The model under review builds one solid part; all positions refer to its coordinate system, in mm. Face numbers are marked on the shaded views. Round coordinates to 2 decimals unless told otherwise and drop trailing zeros. Loops run counter-clockwise (first coordinate to the right, second up) from the corner with the lowest first, then second, coordinate; pieces in that order, holes last. Notation, with made-up numbers: M 35.25,3.5 L 62.25,3.5 A35 cw 62.25,42.5 Z; hole C -7,-30.75 d2. An arc over 180 degrees is marked long. One line per question, with ' | ' between items.
from build123d import *

# Parameters (mm, degrees)
ESBO_O1_R                = 5.25
RESSALTO_EXTRUS_O1_DEPTH = 28.2
ESBO_O1_5_R              = 5
RESSALTO_EXTRUS_O3_DEPTH = 22
RESSALTO_EXTRUS_O4_DEPTH = 27.5
RESSALTO_EXTRUS_O5_DEPTH = 27.5
CORTE_EXTRUS_O3_DEPTH    = 153.972464187
ESBO_O3_R                = 2
CORTE_EXTRUS_O4_DEPTH    = 161.384600668


with BuildPart() as part:
    # Esbo_o1 → Ressalto-extrus_o1 (new, symmetric)
    with BuildSketch(Plane.XY):
        Circle(ESBO_O1_R)
    extrude(amount=RESSALTO_EXTRUS_O1_DEPTH, both=True)

    # Esbo_o1_7 → Ressalto-extrus_o4 (add, symmetric)
    with BuildSketch(Plane.XY):
        with BuildLine():
            Line((60, 5.000779295), (1.598344907, 5.000779295))
            ThreePointArc((1.598344907, 5.000779295), (4.239918087, 3.096061146), (5.25, 0))
            ThreePointArc((5.25, 0), (4.239918087, -3.096061146), (1.598344907, -5.000779295))
            Line((1.598344907, -5.000779295), (60, -5.000779295))
            Line((60, -5.000779295), (60, 5.000779295))
        make_face()
    extrude(amount=RESSALTO_EXTRUS_O4_DEPTH, both=True)



with BuildPart() as body_2:
    # Esbo_o1_5 → Ressalto-extrus_o3 (new, symmetric)
    with BuildSketch(Plane.XY):
        with Locations((145, 1.500779295)):
            Circle(ESBO_O1_5_R)
    extrude(amount=RESSALTO_EXTRUS_O3_DEPTH, both=True)


with BuildPart() as part_1:
    add(part.part)

    add(body_2.part)  # Ressalto-extrus_o5 merges body 2
    # Esbo_o1_8 → Ressalto-extrus_o5 (add, symmetric)
    with BuildSketch(Plane.XY):
        with BuildLine():
            Line((144.911732622, 6.500000121), (60, 5.000779295))
            Line((60, 5.000779295), (60, -5.000779295))
            Line((60, -5.000779295), (145.088267378, -3.498441531))
            ThreePointArc((145.088267378, -3.498441531), (140.000779174, 1.412511917), (144.911732622, 6.500000121))
        make_face()
    extrude(amount=RESSALTO_EXTRUS_O5_DEPTH, both=True)

    # Esbo_o2 → Corte-extrus_o3 (cut, through all)
    with BuildSketch(Plane(origin=(-0.069568666, 3.940177355, 0), x_dir=(0.9998441652583014, 0.01765347554818762, 0), z_dir=(-0.017653475548187615, 0.9998441652583013, 0))):
        Polygon((60.078931051, -27.5), (145.003897933, -22), (145.003897933, -27.5), align=None)
        Polygon((60.078931051, 27.5), (145.003897933, 22), (145.003897933, 27.5), align=None)
    extrude(amount=-CORTE_EXTRUS_O3_DEPTH, mode=Mode.SUBTRACT)

    # Esbo_o3 → Corte-extrus_o4 (cut, through all)
    with BuildSketch(Plane.XY.offset(28.2)):
        Circle(ESBO_O3_R)
    extrude(amount=-CORTE_EXTRUS_O4_DEPTH, mode=Mode.SUBTRACT)


solid = part_1.part
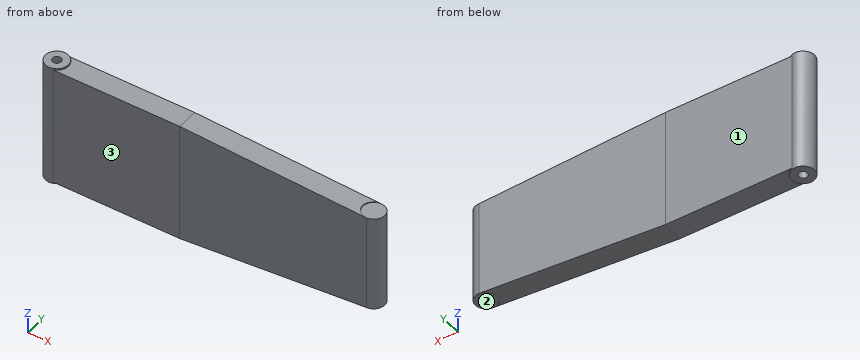
1) Mouldability with a two-part tool opening along Y and no side actions: class the marked faces 1, 2 and 3 as +Y half, -Y half, draft (parallel to the pull), parting line (faces both ways), or undercut.
Output values:
face 1: +Y half | face 2: undercut | face 3: -Y half
2) Insertion check: P1, Ø10, axis at x = 118, z = 11.5, coming from the +Y side; P2, Ø1, axis at x = 40, y = -2, coming from the +Z side; P3, Ø3, axis at y = -3, z = 4.5, coming from the -X side; P4, Ø3.5, axis at x = 0, y = 0, coming from the -Z side. Each pin has a flat end and moves straight along its axis. Give the tip position at first contact, or say it passes through.
Output values:
P1: stops at y = 6.11 | P2: stops at z = 27.5 | P3: stops at x = -5.03 | P4: passes through
3) Add section B-B on x = 0. State the section outline as (y, z) points.
Output values:
outline: M -5.25,-28.2 L -2,-28.2 L -2,28.2 L -5.25,28.2 Z; M 2,-28.2 L 5.25,-28.2 L 5.25,28.2 L 2,28.2 Z
4) Add section D-D on z = -24.5. State the section outline as (x, y) points.
Output values:
outline: M 1.6,-5 L 60,-5 L 106.49,-4.18 L 106.32,5.82 L 60,5 L 1.6,5 A5.25 ccw long Z; hole C 0,0 d4
5) Add section C-C on y = 0. State the section outline as (x, z) points.
Output values:
outline: M -5.25,-28.2 L -2,-28.2 L -2,28.2 L -5.25,28.2 Z; M 2,-28.2 L 5.25,-28.2 L 5.25,-27.5 L 60.09,-27.5 L 140.23,-22.31 L 140.23,-22 L 149.77,-22 L 149.77,22 L 140.23,22 L 140.23,22.31 L 60.09,27.5 L 5.25,27.5 L 5.25,28.2 L 2,28.2 Z
6) Add section A-A on z = 20.5. State the section outline as (x, y) points.
Output values:
outline: M 1.6,-5 L 60,-5 L 145.09,-3.5 A5 ccw 144.91,6.5 L 60,5 L 1.6,5 A5.25 ccw long Z; hole C 0,0 d4
7) For line 1 (Y direction, x = 0, z = 8.5); line 2 (Y direction, x = 19, z = 11.5); line 3 (Z direction, x = 23, y = -1.5), list the stretches that pass through material, from the lowest coordinate up.
Output values:
line 1: y = -5.25 to -2, 2 to 5.25 | line 2: y = -5 to 5 | line 3: z = -27.5 to 27.5
